Verification items for the finished model (mm, model axes). Face numbers are marked on the shaded views. A direction names the side the tool comes from. Round coordinates to 2 decimals unless told otherwise and drop trailing zeros. Write each loop counter-clockwise with the first axis right and the second up, starting at its lowest first coordinate (ties: lowest second). Pieces come first, ordered by that corner, then holes.
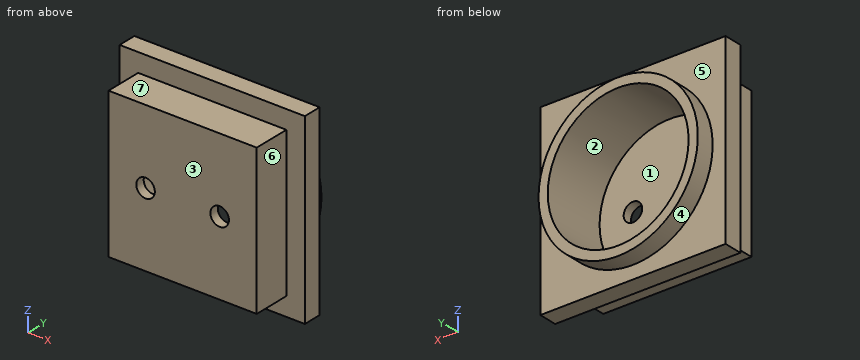
from build123d import *

# Parameters (mm, degrees)
CROQUIS1_W              = 50
CROQUIS1_H              = 50
SALIENTE_EXTRUIR1_DEPTH = 5
CROQUIS2_R              = 21.5
SALIENTE_EXTRUIR2_DEPTH = 5
CROQUIS4_W              = 40
CROQUIS4_H              = 40
SALIENTE_EXTRUIR3_DEPTH = 10
CROQUIS3_R              = 19
CORTAR_EXTRUIR1_DEPTH   = 17.5
CROQUIS5_R              = 2.5
CORTAR_EXTRUIR2_DEPTH   = 3.5


with BuildPart() as part:
    # Croquis1 → Saliente-Extruir1 (new body)
    with BuildSketch(Plane(origin=(0, 0, 0), x_dir=(1, 0, 0), z_dir=(0, 1, 0))):
        Rectangle(CROQUIS1_W, CROQUIS1_H)
    extrude(amount=SALIENTE_EXTRUIR1_DEPTH)

    # Croquis2 → Saliente-Extruir2 (add)
    with BuildSketch(Plane(origin=(0, 5, 0), x_dir=(1, 0, 0), z_dir=(0, 1, 0))):
        Circle(CROQUIS2_R)
    extrude(amount=SALIENTE_EXTRUIR2_DEPTH)

    # Croquis4 → Saliente-Extruir3 (add)
    with BuildSketch(Plane.XZ):
        Rectangle(CROQUIS4_W, CROQUIS4_H)
    extrude(amount=SALIENTE_EXTRUIR3_DEPTH)

    # Croquis3 → Cortar-Extruir1 (cut)
    with BuildSketch(Plane(origin=(0, 10, 0), x_dir=(1, 0, 0), z_dir=(0, 1, 0))):
        Circle(CROQUIS3_R)
    extrude(amount=-CORTAR_EXTRUIR1_DEPTH, mode=Mode.SUBTRACT)

    # Croquis5 → Cortar-Extruir2 (cut, through all)
    with BuildSketch(Plane(origin=(0, -7.5, 0), x_dir=(1, 0, 0), z_dir=(0, 1, 0))):
        with Locations((10, 0)):
            Circle(CROQUIS5_R)
        with Locations((-10, 0)):
            Circle(CROQUIS5_R)
    extrude(amount=-CORTAR_EXTRUIR2_DEPTH, mode=Mode.SUBTRACT)


solid = part.part
Q1. Sectioned sample at A-A (y = -1.75). Enter the section's corners in (x, z).
Recorded:
outline: (-20, -20) - (20, -20) - (20, 20) - (-20, 20) - close; hole circle Ø38 at (0, 0)
Q2. Release check for a two-part mould opening along Z. For the marked faces 1, 2, 3 and 4 record: released by +Z, released by -Z, zero draft, split by the parting line, or undercut.
Recorded:
face 1: undercut
face 2: undercut
face 3: zero draft
face 4: split by the parting line
Q3. Sectioned sample at B-B (x = 0). Enter the section's corners in (y, z), plus the area to 3 significant figures.
Recorded:
outline: (-10, -20) - (0, -20) - (0, -25) - (5, -25) - (5, -21.5) - (10, -21.5) - (10, -19) - (-7.5, -19) - (-7.5, 19) - (10, 19) - (10, 21.5) - (5, 21.5) - (5, 25) - (0, 25) - (0, 20) - (-10, 20) - close
area: 200 mm2
Q4. Material ranges on line 1 along X through (y, z) = (-9.3, 0); line 2 along Z through (x, y) = (0, -3.25); line 3 along Z through (x, y) = (-10, -9.1), recorded low to high.
Recorded:
line 1: x = -20 to -12.5, -7.5 to 7.5, 12.5 to 20
line 2: z = -20 to -19, 19 to 20
line 3: z = -20 to -2.5, 2.5 to 20
Q5. Sectioned sample at C-C (x = -10). Enter the section's corners in (y, z), plus the area to 3 significant figures.
Recorded:
outline: (-10, -20) - (0, -20) - (0, -25) - (5, -25) - (5, -19.03) - (10, -19.03) - (10, -16.16) - (-7.5, -16.16) - (-7.5, -2.5) - (-10, -2.5) - close; (-10, 2.5) - (-7.5, 2.5) - (-7.5, 16.16) - (10, 16.16) - (10, 19.03) - (5, 19.03) - (5, 25) - (0, 25) - (0, 20) - (-10, 20) - close
area: 262 mm2
Q6. Tool access check on the marked faces 5, 6 and 7. Record the directions out of +Z, -Z, +X, -X, +Y, -Y that give a thin tool (end or side, any length) a straight path to the whole face; none if there is none.
Recorded:
face 5: +Y
face 6: +Z, -Z, +X, -Y
face 7: +Z, +X, -X, -Y
Q7. Depth check by flat-ended pin: P1, Ø5, axis at x = -5.5, y = -5.5, coming from the +Z side; P2, Ø1.5, axis at x = 20, z = 12, coming from the +Y side; P3, Ø5, axis at y = -5.5, z = 0.5, coming from the +X side. Enter the tip coordinate at first touch or a pass-through.
Recorded:
P1: stops at z = 20
P2: stops at y = 5
P3: stops at x = 20
Q8. Sectioned sample at D-D (z = -18). Enter the section's corners in (x, y), plus the area to 3 significant figures.
Recorded:
outline: (-25, 0) - (-20, 0) - (-20, -10) - (20, -10) - (20, 0) - (25, 0) - (25, 5) - (11.76, 5) - (11.76, 10) - (6.08, 10) - (6.08, -7.5) - (-6.08, -7.5) - (-6.08, 10) - (-11.76, 10) - (-11.76, 5) - (-25, 5) - close
area: 555 mm2
